```python
from build123d import *

# Parameters (mm, degrees)
GUARD_BASE_R     = 25
GUARD_DEPTH      = 5
AXLE_HOLE_BASE_R = 15.75
AXLE_HOLE_DEPTH  = 6


with BuildPart() as part:
    # Guard base → Guard (new body)
    with BuildSketch(Plane.XY):
        Circle(GUARD_BASE_R)
    extrude(amount=GUARD_DEPTH)

    # Axle hole base → Axle hole (cut, through all)
    with BuildSketch(Plane.XY.offset(5)):
        Circle(AXLE_HOLE_BASE_R)
    extrude(amount=-AXLE_HOLE_DEPTH, mode=Mode.SUBTRACT)

    # Mate ring room base → Mate ring room (revolve, cut)
    with BuildSketch(Plane(origin=(0, 0, 0), x_dir=(1, 0, 0), z_dir=(0, 1, 0))):
        Polygon((15.75, -5), (16.5, -5), (15.75, -4.25), align=None)
        Polygon((15.75, 0), (16.5, 0), (15.75, -0.75), align=None)
    revolve(axis=Axis((0, 0, 0), (0, 0, -1)), mode=Mode.SUBTRACT)


solid = part.part
```
The model under review builds one solid part; all positions refer to its coordinate system, in mm. Round coordinates to 2 decimals unless told otherwise and drop trailing zeros. Loops run counter-clockwise (first coordinate to the right, second up) from the corner with the lowest first, then second, coordinate; pieces in that order, holes last. Notation, with made-up numbers: (-31.75, 15) -> (0.25, 15) arc R17 ccw to (0.25, 35) -> close; hole circle Ø10 at (-20, 59.25). An arc over 180 degrees is marked (long way). Answer as a JSON object with one key per item and string values. Group by question number.
1) We need section A-A on x = 0. Write out the cut boundary in (y, z), then the cut area to 3 significant figures.
2) We need section C-C on z = 3.4. Write out the cut boundary in (x, y).
3) For line 1 (Y direction, x = 0, z = 2.5); line 2 (Y direction, x = 3, z = 2.05); line 3 (X direction, y = 3.5, z = 1.8), list the stretches that pass through material, from the lowest coordinate up. Write a range as [from, to].
4) Mouldability with a two-part tool opening along Y and no side actions: class faces 1 (the face through (-2.05, 15.616, 2.524)), 2 (the face through (5, -16, 0)), 3 (the face through (23.846, 7.509, 2.465)) as released by +Y, released by -Y, zero draft, split by the parting line, or undercut.
5) We need section D-D on y = 20. Write out the cut boundary in (x, z).
6) For pin 1 Ø1 at (y, z) = (-11, 3.5) entering from +X; pin 2 Ø6 at (x, y) = (-15, 3) entering from -Z; pin 3 Ø2 at (x, z) = (6.5, 4) entering from -Y; pin 4 Ø2 at (y, z) = (-1.5, 4) entering from -X (3 decimals), all flat-tipped, find the tip position at first contact; note any pin that passes through.
Result set:
{
 "1": {"outline": "(-25, 0) -> (-16.5, 0) -> (-15.75, 0.75) -> (-15.75, 4.25) -> (-16.5, 5) -> (-25, 5) -> close; (15.75, 0.75) -> (16.5, 0) -> (25, 0) -> (25, 5) -> (16.5, 5) -> (15.75, 4.25) -> close", "area": "91.4 mm²"},
 "2": {"outline": "circle Ø50 at (0, 0); hole circle Ø31.5 at (0, 0)"},
 "3": {"line 1": "[-25, -15.75], [15.75, 25]", "line 2": "[-24.82, -15.46], [15.46, 24.82]", "line 3": "[-24.75, -15.36], [15.36, 24.75]"},
 "4": {"face 1": "undercut", "face 2": "zero draft", "face 3": "split by the parting line"},
 "5": {"outline": "(-15, 0) -> (15, 0) -> (15, 5) -> (-15, 5) -> close"},
 "6": {"pin 1": "x = 22.69", "pin 2": "z = 0", "pin 3": "y = -24.39", "pin 4": "x = -24.995"}
}
